Model file for the job. Use its own axes, mm. A direction names the side the tool comes from. Coordinates: 2 decimals unless noted, no trailing zeros. Order: outer loops, then holes, each group sorted by start corner. A loop starts at its lowest first (then second) coordinate and runs counter-clockwise, first axis right, second up. Notation, with made-up numbers: (65, 31.25) - (111, 31.25) arc R8 ccw to (111, 43.25) - close; hole circle Ø6 at (13.5, 27). An arc over 180 degrees is marked (long way). Put each result on its own line as item: value. Start each with the question number.
```python
from build123d import *

# Parameters (mm, degrees)
SKETCH1_R           = 241.3
BOSS_EXTRUDE1_DEPTH = 5080
SKETCH2_R           = 762
BOSS_EXTRUDE3_DEPTH = 1778
CUT_EXTRUDE2_START  = -1778
CUT_EXTRUDE2_DEPTH  = 5252.397760119
CIRPATTERN1_COUNT   = 3
SCALE1_SCALE        = 0.02


with BuildPart() as part:
    # Sketch1 → Boss-Extrude1 (new body)
    with BuildSketch(Plane(origin=(0, 0, 0), x_dir=(1, 0, 0), z_dir=(0, 1, 0))):
        with Locations(Location((0, 0, 0), (0, 0, 90))):
            Circle(SKETCH1_R)
    extrude(amount=BOSS_EXTRUDE1_DEPTH)

    # Sketch2 → Boss-Extrude3 (add)
    with BuildSketch(Plane.XZ):
        with Locations(Location((0, 0, 0), (0, 0, 270))):
            Circle(SKETCH2_R)
    extrude(amount=-BOSS_EXTRUDE3_DEPTH)

    # Sketch4 → Cut-Extrude2 (cut)
    with BuildSketch(Plane(origin=(0, 1778, 0), x_dir=(1, 0, 0), z_dir=(0, 1, 0)).offset(CUT_EXTRUDE2_START)):
        with BuildLine():
            Line((2450.032308946, 3662.965924128), (356.689294384, 673.362270455))
            Line((356.689294384, 673.362270455), (50.425576786, 235.97235263))
            ThreePointArc((50.425576786, 235.97235263), (0, 241.3), (-50.425576786, 235.97235263))
            Line((-50.425576786, 235.97235263), (-356.689294384, 673.362270455))
            Line((-356.689294384, 673.362270455), (-2450.032308946, 3662.965924128))
            Line((-2450.032308946, 3662.965924128), (-2450.032308946, 10962.230265875))
            Line((-2450.032308946, 10962.230265875), (2450.032308946, 10962.230265875))
            Line((2450.032308946, 10962.230265875), (2450.032308946, 3662.965924128))
        make_face()
    cut_extrude2 = extrude(amount=CUT_EXTRUDE2_DEPTH, mode=Mode.SUBTRACT)

    # CirPattern1: Cut-Extrude2 ×3 about axis
    cirpattern1_axis = Axis((0, 5080, 0), (0, -1, 0))
    for i in range(1, CIRPATTERN1_COUNT):
        add(cut_extrude2.rotate(cirpattern1_axis, i * 360 / CIRPATTERN1_COUNT), mode=Mode.SUBTRACT)


with BuildPart() as part_1:
    # Scale1: scaled about (0, 1463.203660293, 0)
    add(part.part.scale(SCALE1_SCALE).moved(Location((0, 1433.939587087, 0))))


solid = part_1.part
```
Item 1: Wall check: line 1 along Z through (x, y) = (-1.5, 1475); line 2 along Y through (x, z) = (6, 12); line 3 along X through (y, z) = (1461.5, -11.25). Give the ranges that are in metal, low to high.
Item 2: 3-axis set-ups, long thin cutter, end or side, ignore diameter. For faces 1 (the face through (0, 1433.94, 1)), 2 (the face through (-5.808, 1451.471, 8.005)), 3 (the face through (4.11, 1451.47, -9.15)), 4 (the face through (5.87, 1451.47, 8.14)): which of +Z, -Z, +X, -X, +Y, -Y reach the whole face in a straight line?
Item 3: Slice it at A-A, the plane z = -11.5. Give the cut face in (x, y).
Item 4: Slice it at D-D, the plane z = -1.5. Give the cut face in (x, y), plus the area to 3 significant figures.
Item 5: Slice it at C-C, the plane x = -2. Give the cut face in (y, z).
Item 6: Slice it at B-B, the plane y = 1467. Give the cut face in (x, z).
Item 7: Flat gauge pins, fed straight in: pin 1 Ø3 at (x, y) = (5.5, 1470) entering from -Z; pin 2 Ø1 at (y, z) = (1464.5, 9.5) entering from +X; pin 3 Ø6 at (x, z) = (-1.5, 8) entering from +Y; pin 4 Ø10 at (y, z) = (1470, 4) entering from -X. Where does each tip first touch, or does it go through?
Item 8: Pull direction X, two halves, no side cores. Call faces 5 (the face through (-4.028, 1451.471, -9.032)), 6 (the face through (0.12, 1451.47, 15.24)), 7 (the face through (-8, 1469.5, -4)): pulls with the +X half, pulls with the -X half, needs draft (parallel to the pull), parting line crosses it, or undercut.
Here are the results:
1. line 1: z = -4.59 to 4.59
1. line 2: y = 1433.94 to 1469.5
1. line 3: x = -10.28 to -5.58, 5.58 to 10.28
2. face 1: +Z, -Z, +X, -X, -Y
2. face 2: -X, +Y, -Y
2. face 3: -Z, +Y, -Y
2. face 4: +X, +Y, -Y
3. outline: (-10, 1433.94) - (-5.76, 1433.94) - (-5.76, 1469.5) - (-10, 1469.5) - close; (5.76, 1433.94) - (10, 1433.94) - (10, 1469.5) - (5.76, 1469.5) - close
4. outline: (-15.17, 1433.94) - (15.17, 1433.94) - (15.17, 1469.5) - (4.59, 1469.5) - (4.59, 1535.54) - (-4.59, 1535.54) - (-4.59, 1469.5) - (-15.17, 1469.5) - close
4. area: 1,680 mm^2
5. outline: (1433.94, -6.14) - (1469.5, -6.14) - (1469.5, -4.39) - (1535.54, -4.39) - (1535.54, 4.39) - (1469.5, 4.39) - (1469.5, 15.11) - (1433.94, 15.11) - close
6. outline: (-15.23, 0.56) arc R15.24 ccw to (-7.13, -13.47) - (-1.01, -4.72) arc R4.83 ccw to (1.01, -4.72) - (7.13, -13.47) arc R15.24 ccw to (15.23, 0.56) - (4.59, 1.49) arc R4.83 ccw to (3.58, 3.23) - (8.1, 12.91) arc R15.24 ccw to (-8.1, 12.91) - (-3.58, 3.23) arc R4.83 ccw to (-4.59, 1.49) - close
7. pin 1: stops at z = -13.15
7. pin 2: stops at x = 6.74
7. pin 3: stops at y = 1469.5
7. pin 4: stops at x = -15.24
8. face 5: undercut
8. face 6: parting line crosses it
8. face 7: needs draft
